Input: dimensioned drawing with shaded views. Units: mm. Origin: part minimum x, y, z. Round coordinates to 2 decimals unless told otherwise and drop trailing zeros. Write each loop counter-clockwise with the first axis right and the second up, starting at its lowest first coordinate (ties: lowest second). Pieces come first, ordered by that corner, then holes. Notation, with made-up numbers: M 31.5,-14.75 L 71.5,-14.75 A29 ccw 71.5,18.25 Z; hole C 61.5,20.5 d3. An arc over 180 degrees is marked long. Answer in a Markdown table with one row per item. Add a question column.
Item 1: Cut plane C-C on y = 0.2. Return loops of the section in (x, z), and give its area (4 significant figures).
Item 2: Material intervals for probe 1 along Z at (x, y) = (4.5, 1.95); probe 2 along Y at (x, z) = (6.25, 6.75), sorted ascending.
Item 3: Cut plane D-D on x = 4.25. Return loops of the section in (y, z).
Item 4: Mould query, pull axis X, two halves, no side actions, for the marked faces 1, 2, 3 and 4. Classes: released by +X, released by -X, zero draft, split by the parting line, or undercut.
Item 5: Contact query for flat-ended pins moving along their axis: pin 1 (0.5 mm diameter, centred on y = 1, z = 5, fed in from -X); pin 2 (0.5 mm diameter, centred on x = 3.5, z = 6, fed in from +Y); pin 3 (1 mm diameter, centred on y = 2, z = 4.5, fed in from +X); pin 4 (0.6 mm diameter, centred on y = 1, z = 4, fed in from +X). Output: stop coordinate, or through.
Item 6: Cut plane A-A on z = 7.5. Return loops of the section in (x, y), and give its area (3 significant figures).
Item 7: Cut plane B-B on x = 6. Return loops of the section in (y, z).
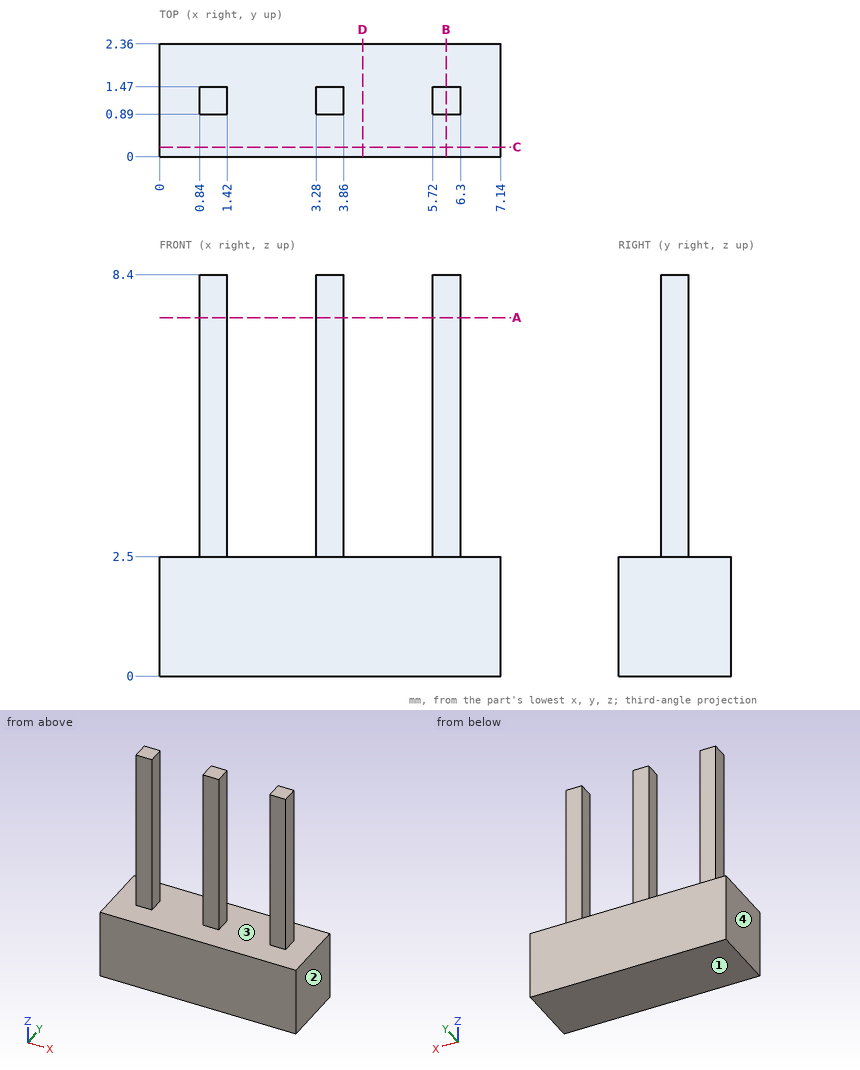
Results below:
| question | item | result |
|---|---|---|
| 1 | outline | M 0,0 L 7.14,0 L 7.14,2.5 L 0,2.5 Z |
| 1 | area | 17.85 mm2 |
| 2 | probe 1 | 0 to 2.5 |
| 2 | probe 2 | 0.89 to 1.47 |
| 3 | outline | M 0,0 L 2.36,0 L 2.36,2.5 L 0,2.5 Z |
| 4 | face 1 | zero draft |
| 4 | face 2 | released by +X |
| 4 | face 3 | undercut |
| 4 | face 4 | released by -X |
| 5 | pin 1 | x = 0.84 |
| 5 | pin 2 | y = 1.47 |
| 5 | pin 3 | through |
| 5 | pin 4 | x = 6.3 |
| 6 | outline | M 0.84,0.89 L 1.42,0.89 L 1.42,1.47 L 0.84,1.47 Z; M 3.28,0.89 L 3.86,0.89 L 3.86,1.47 L 3.28,1.47 Z; M 5.72,0.89 L 6.3,0.89 L 6.3,1.47 L 5.72,1.47 Z |
| 6 | area | 1.01 mm2 |
| 7 | outline | M 0,0 L 2.36,0 L 2.36,2.5 L 1.47,2.5 L 1.47,8.4 L 0.89,8.4 L 0.89,2.5 L 0,2.5 Z |
